from build123d import *

# Parameters (mm, degrees)
SKETCH1_R           = 22
BOSS_EXTRUDE2_DEPTH = 2
SKETCH4_R           = 20.5
BOSS_EXTRUDE3_DEPTH = 1
SKETCH5_R           = 19.5
CUT_EXTRUDE1_DEPTH  = 32.256999216


with BuildPart() as part:
    # Sketch1 → Boss-Extrude2 (new body)
    with BuildSketch(Plane.XY):
        Circle(SKETCH1_R)
    extrude(amount=BOSS_EXTRUDE2_DEPTH)

    # Sketch4 → Boss-Extrude3 (add)
    with BuildSketch(Plane(origin=(0, 0, 0), x_dir=(-1, 0, 0), z_dir=(0, 0, -1))):
        Circle(SKETCH4_R)
    extrude(amount=BOSS_EXTRUDE3_DEPTH)

    # Sketch5 → Cut-Extrude1 (cut, through all)
    with BuildSketch(Plane(origin=(0, 0, -1), x_dir=(-1, 0, 0), z_dir=(0, 0, -1))):
        Circle(SKETCH5_R)
    extrude(amount=-CUT_EXTRUDE1_DEPTH, mode=Mode.SUBTRACT)


solid = part.part
The listing builds one solid part. Answer for the finished solid, in the listing's coordinates (mm). Give positions to 0.01 mm unless a question says otherwise; leave off trailing zeros. Write each loop counter-clockwise with the first axis right and the second up, starting at its lowest first coordinate (ties: lowest second). Pieces come first, ordered by that corner, then holes.
Item 1: Flat-ended cylindrical pins translate along their axes: P1, Ø8, axis at x = 15, y = 3, coming from the -Z side; P2, Ø22, axis at x = -2.5, y = 9.5, coming from the -Z side; P3, Ø1.5, axis at x = -7, z = -0.5, coming from the -Y side. Find the tip coordinate at first contact, or state that the pin passes through.
Item 2: Section A-A, the plane x = 0 is taken. Write down the section's boundary in (y, z), plus the area to 3 significant figures.
Item 3: Section C-C, the plane z = 0.8 is taken. Write down the section's boundary in (x, y).
Item 4: Find the intervals of material crossed by line 1 along Y through (x, z) = (0, -0.05); line 2 along Y through (x, z) = (0, 0.45); line 3 along X through (y, z) = (-13, 1.05), in increasing order.
Item 5: Determine the mould class of faces 1 (the cylindrical face through (4.444, -20.013, -0.493)), 2 (the cylindrical face through (2.539, 19.334, 0.479)), 3 (the flat face through (15, -15, 0)) for opening direction X: released by +X, released by -X, zero draft, split by the parting line, or undercut.
Completed:
1. P1: passes through
1. P2: stops at z = -1
1. P3: stops at y = -21.04
2. outline: (-22, 0) - (-20.5, 0) - (-20.5, -1) - (-19.5, -1) - (-19.5, 2) - (-22, 2) - close; (19.5, -1) - (20.5, -1) - (20.5, 0) - (22, 0) - (22, 2) - (19.5, 2) - close
2. area: 12.0 mm2
3. outline: circle Ø44 at (0, 0); hole circle Ø39 at (0, 0)
4. line 1: y = -20.5 to -19.5, 19.5 to 20.5
4. line 2: y = -22 to -19.5, 19.5 to 22
4. line 3: x = -17.75 to -14.53, 14.53 to 17.75
5. face 1: split by the parting line
5. face 2: undercut
5. face 3: zero draft
